Verification items for this drawing (mm, ordinates from the low corner). A direction names the side the tool comes from. Coordinates: 2 decimals unless noted, no trailing zeros. Loops run counter-clockwise (first coordinate to the right, second up) from the corner with the lowest first, then second, coordinate; pieces in that order, holes last. Notation, with made-up numbers: (-34.5, -8) - (18.5, -8) arc R14 ccw to (18.5, 18) - close; hole circle Ø7 at (-1, 76.5). An arc over 180 degrees is marked (long way). Write each question's results on one line, items separated by ' | '. Start each with the question number.
(1) Access from +Z, -Z, +X, -X, +Y, -Y to the whole of each face (thin tool, end or side, straight path). Record for the marked faces 1 and 2.
(2) Go/stop test with flat-tipped pins: pin 1 Ø1.5 at (x, z) = (46, 47) entering from +Y; pin 2 Ø12 at (x, z) = (80, 45.5) entering from -Y. Record where each tip stops, or that it passes through.
(3) Mould release check, pull along X, two halves, no side actions. Record for the marked faces 3, 4 and 5: pulls with the +X half, pulls with the -X half, needs draft (parallel to the pull), parting line crosses it, or undercut.
(4) Sectioned sample at A-A (z = 83.5). Enter the section's corners in (x, y).
(5) Material ranges on probe 1 along Z at (x, y) = (58.5, 44); probe 2 along X at (y, z) = (25, 48); probe 3 along Y at (x, z) = (56.5, 74), recorded low to high.
(6) Sectioned sample at C-C (x = 59.5). Enter the section's corners in (y, z), plus the area to 3 significant figures.
(7) Sectioned sample at B-B (y = 19.5). Enter the section's corners in (x, z).
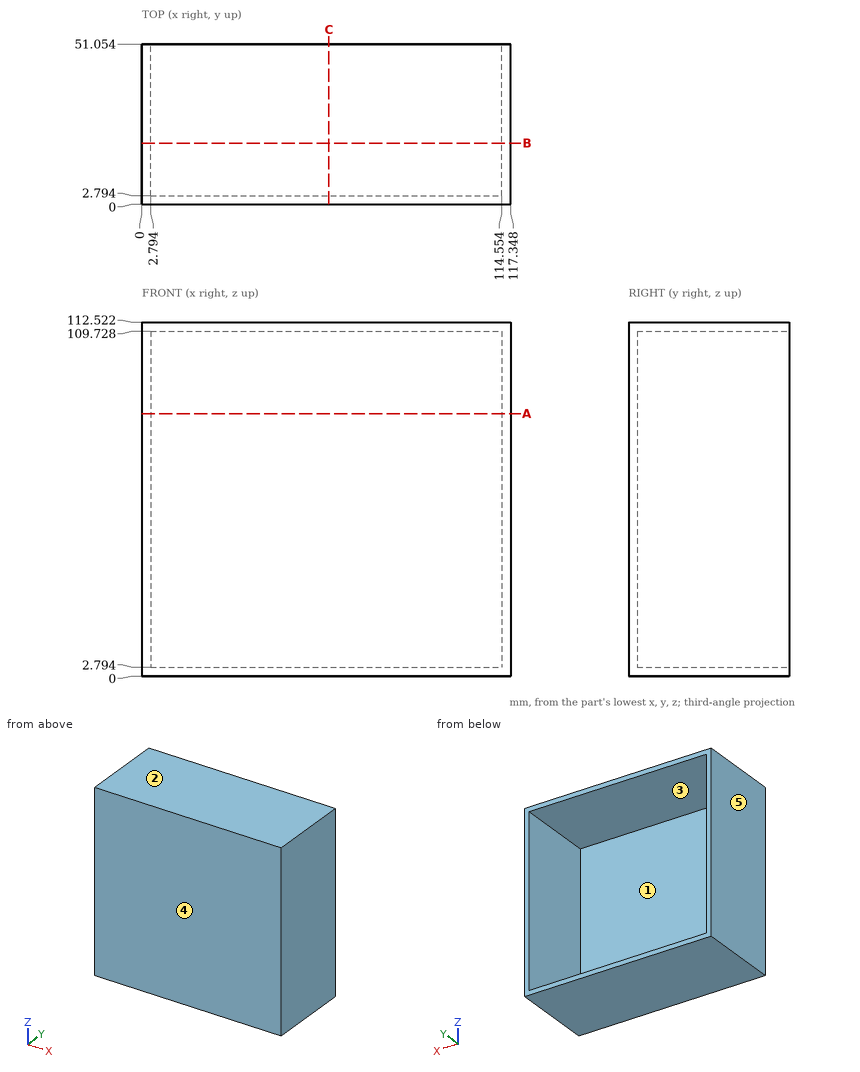
Outcome:
1) face 1: +Y | face 2: +Z, +X, -X, +Y, -Y
2) pin 1: stops at y = 2.79 | pin 2: stops at y = 0
3) face 3: undercut | face 4: needs draft | face 5: pulls with the -X half
4) outline: (0, 0) - (117.35, 0) - (117.35, 51.05) - (114.55, 51.05) - (114.55, 2.79) - (2.79, 2.79) - (2.79, 51.05) - (0, 51.05) - close
5) probe 1: z = 0 to 2.79, 109.73 to 112.52 | probe 2: x = 0 to 2.79, 114.55 to 117.35 | probe 3: y = 0 to 2.79
6) outline: (0, 0) - (51.05, 0) - (51.05, 2.79) - (2.79, 2.79) - (2.79, 109.73) - (51.05, 109.73) - (51.05, 112.52) - (0, 112.52) - close | area: 584 mm2
7) outline: (0, 0) - (117.35, 0) - (117.35, 112.52) - (0, 112.52) - close; hole (2.79, 2.79) - (114.55, 2.79) - (114.55, 109.73) - (2.79, 109.73) - close
